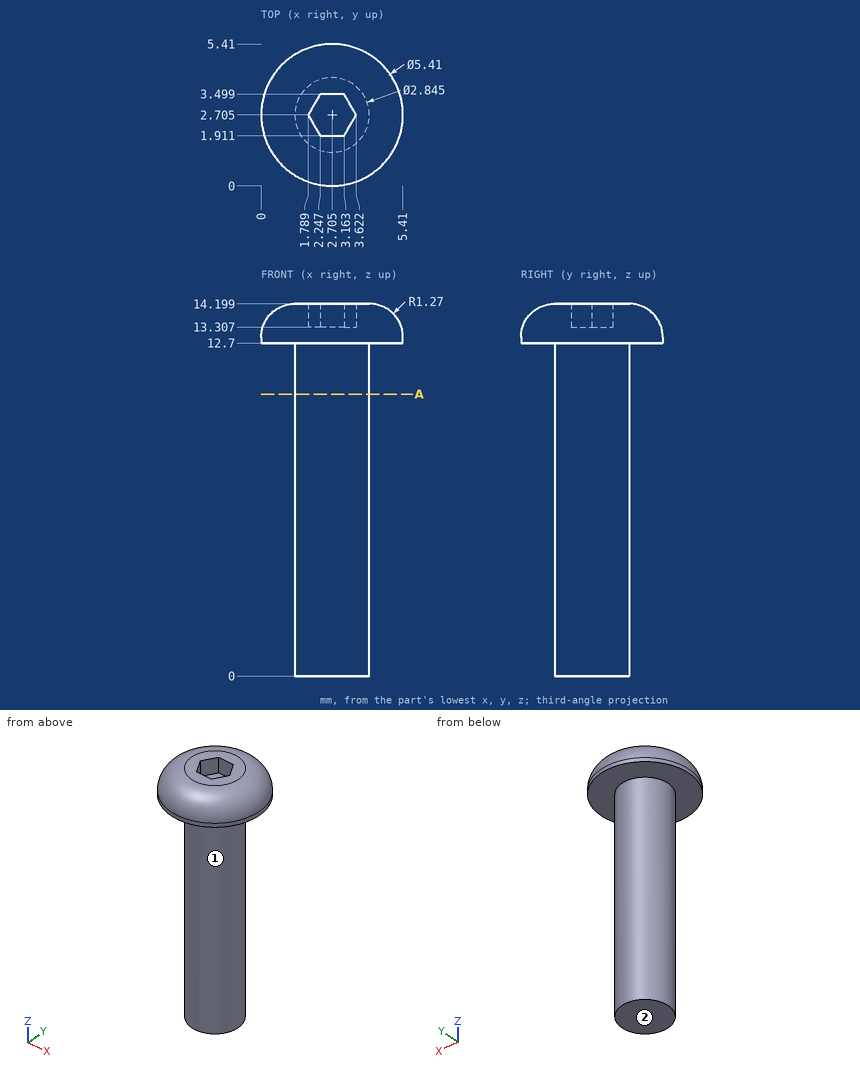
Geometry: see drawing. Coordinates: mm, zero at the bounding-box minimum. A direction names the side the tool comes from. Round coordinates to 2 decimals unless told otherwise and drop trailing zeros. Write each loop counter-clockwise with the first axis right and the second up, starting at its lowest first coordinate (ties: lowest second). Pieces come first, ordered by that corner, then holes. Notation, with made-up numbers: (47.5, 28) - (74.5, 28) arc R13 ccw to (74.5, 36) - close; hole circle Ø4 at (-10.5, -36). An arc over 180 degrees is marked (long way). Use CSV: the item, a comma, the result in double quotes. Start each with the question number.
(1) Set-up query: the marked faces 1 and 2. Return all of +Z, -Z, +X, -X, +Y, -Y with unobstructed straight access to the full face (end or side cutting, diameter ignored); none if empty.
(2) First-contact query: pin 1 Ø3 at (y, z) = (4, 9) entering from -X; pin 2 Ø1 at (y, z) = (4, 4.5) entering from -X (1 decimal); pin 3 Ø0.5 at (x, y) = (2.5, 3) entering from +Z. Flat tips, straight axial feed; report the tip coordinate or a pass-through.
(3) Cut plane A-A, the plane z = 10.75. Return loops of the section in (x, y) (1 decimal).
(4) Material intervals for probe 1 along Y at (x, z) = (2.6, 9.25); probe 2 along Y at (x, z) = (2.1, 1.75); probe 3 along Z at (x, y) = (3.3, 0.5) (1 decimal), sorted ascending. Write a range as [from, to].
Geometry says:
1,face 1,"-Z"
1,face 2,"-Z, +X, -X, +Y, -Y"
2,pin 1,"x = 1.28"
2,pin 2,"x = 1.5"
2,pin 3,"z = 13.31"
3,outline,"circle Ø2.8 at (2.7, 2.7)"
4,probe 1,"[1.29, 4.12]"
4,probe 2,"[1.42, 3.99]"
4,probe 3,"[12.7, 13.9]"
